```python
from build123d import *

# Parameters (mm, degrees)
SKETCH1_R                      = 3.175
BOSS_EXTRUDE1_DEPTH            = 19.05
CUT_EXTRUDE1_REACH             = 5.175
SKETCH2_R                      = 1.4986
CUT_EXTRUDE1_DIRECTION_2_DEPTH = 19.05


with BuildPart() as part:
    # Sketch1 → Boss-Extrude1 (new body)
    with BuildSketch(Plane(origin=(0, 0, 0), x_dir=(1, 0, 0), z_dir=(0, 1, 0))):
        Circle(SKETCH1_R)
    extrude(amount=BOSS_EXTRUDE1_DEPTH)

    # Sketch2 → Cut-Extrude1 (cut, up to next)
    with BuildSketch(Plane.XY, mode=Mode.PRIVATE) as cut_extrude1_sk1:
        with Locations((0, 9.525)):
            Circle(SKETCH2_R)
    cut_extrude1_tool1 = extrude(cut_extrude1_sk1.sketch, amount=-CUT_EXTRUDE1_REACH, mode=Mode.PRIVATE) & part.part
    add(cut_extrude1_tool1.solids().sort_by_distance((0, 9.525, 0))[0], mode=Mode.SUBTRACT)

    # Sketch2 → Cut-Extrude1 direction 2 (cut)
    with BuildSketch(Plane.XY):
        with Locations((0, 9.525)):
            Circle(SKETCH2_R)
    extrude(amount=CUT_EXTRUDE1_DIRECTION_2_DEPTH, mode=Mode.SUBTRACT)


solid = part.part
```
Geometry: final body of the model. Coordinates: model frame, mm. Round coordinates to 2 decimals unless told otherwise and drop trailing zeros. Loops run counter-clockwise (first coordinate to the right, second up) from the corner with the lowest first, then second, coordinate; pieces in that order, holes last.
Item 1: Section A-A, the plane x = 0. Output: boundary loops of the cut face in (y, z) (3 decimals).
Checked values:
outline: (0, -3.175) - (8.026, -3.175) - (8.026, 3.175) - (0, 3.175) - close; (11.024, -3.175) - (19.05, -3.175) - (19.05, 3.175) - (11.024, 3.175) - close
Item 2: Section D-D, the plane y = 8.25. Output: boundary loops of the cut face in (x, z) (3 decimals), plus the area to 3 significant figures.
Checked values:
outline: (-0.788, -3.076) - (-0.788, 3.076) arc R3.175 ccw to start; (0.788, -3.076) arc R3.175 ccw to (0.788, 3.076) - close
area: 21.8 mm2
Item 3: Section B-B, the plane z = -1.25. Output: boundary loops of the cut face in (x, y) (3 decimals).
Checked values:
outline: (-2.919, 0) - (2.919, 0) - (2.919, 19.05) - (-2.919, 19.05) - close; hole circle Ø2.997 at (0, 9.525)
Item 4: Line query: L1, parallel to Y at x = 0, z = 0; L2, parallel to X at y = 10, z = 2.5; L3, parallel to X at y = 10, z = -1. Output: solid intervals per line, ascending.
Checked values:
L1: y = 0 to 8.03, 11.02 to 19.05
L2: x = -1.96 to -1.42, 1.42 to 1.96
L3: x = -3.01 to -1.42, 1.42 to 3.01
Item 5: Section C-C, the plane y = 6. Output: boundary loops of the cut face in (x, z) (3 decimals), plus the area to 3 significant figures.
Checked values:
outline: circle Ø6.35 at (0, 0)
area: 31.7 mm2
Item 6: Mould query, pull axis Y, two halves, no side actions, for faces 1 (the cylindrical face through (1.707, 9.392, -2.677)), 2 (the flat face through (0, 19.05, 0)), 3 (the cylindrical face through (-1.497, 9.591, 0.045)). Classes: released by +Y, released by -Y, zero draft, split by the parting line, or undercut.
Checked values:
face 1: zero draft
face 2: released by +Y
face 3: undercut
